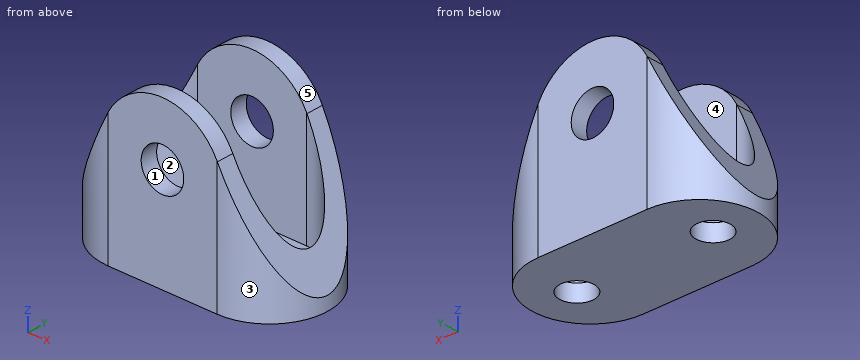
```python
from build123d import *

# Parameters (mm, degrees)
SKETCH1_W          = 44.45
SKETCH1_H          = 31.75
BILLET_DEPTH       = 21.59
SKETCH2_R          = 3.96875
MILL_CUT_1_DEPTH   = 22.59
CUT_EXTRUDE1_DEPTH = 27.305
CUT_EXTRUDE2_DEPTH = 31.48
SKETCH9_R          = 3.175
HOLES_DEPTH        = 4.1750001


with BuildPart() as part:
    # Sketch1 → Billet (new body)
    with BuildSketch(Plane(origin=(0, 0, 0), x_dir=(1, 0, 0), z_dir=(0, 1, 0))):
        Rectangle(SKETCH1_W, SKETCH1_H)
    extrude(amount=BILLET_DEPTH)

    # Sketch2 → Mill Cut 1 (cut, through all)
    with BuildSketch(Plane(origin=(0, 21.59, 0), x_dir=(1, 0, 0), z_dir=(0, 1, 0))):
        with Locations((0, -3.175)):
            Circle(SKETCH2_R)
        with BuildLine():
            Line((-10.236684927, -8.259799082), (-22.225, 15.875))
            Line((-22.225, 15.875), (-22.225, -15.875))
            Line((-22.225, -15.875), (22.225, -15.875))
            Line((22.225, -15.875), (22.225, 15.875))
            Line((22.225, 15.875), (10.236684927, -8.259799082))
            ThreePointArc((10.236684927, -8.259799082), (0, -14.605), (-10.236684927, -8.259799082))
        make_face()
    extrude(amount=-MILL_CUT_1_DEPTH, mode=Mode.SUBTRACT)

    # Sketch6 → Cut-Extrude1 (cut)
    with BuildSketch(Plane(origin=(0, 21.59, 14.605), x_dir=(1, 0, 0), z_dir=(0, 0, 1))):
        with BuildLine():
            Line((-10.16, -3.175), (10.16, -3.175))
            ThreePointArc((10.16, -3.175), (17.78, -10.795), (10.16, -18.415))
            Line((10.16, -18.415), (-10.16, -18.415))
            ThreePointArc((-10.16, -18.415), (-17.78, -10.795), (-10.16, -3.175))
        make_face()
    extrude(amount=-CUT_EXTRUDE1_DEPTH, mode=Mode.SUBTRACT)

    # Sketch8 → Cut-Extrude2 (cut, through all)
    with BuildSketch(Plane(origin=(0, 21.59, 14.605), x_dir=(1, 0, 0), z_dir=(0, 0, 1))):
        with BuildLine():
            Line((-10.16, -21.59), (-60.96, -21.59))
            Line((-60.96, -21.59), (-60.96, 0))
            Line((-60.96, 0), (-10.16, 0))
            ThreePointArc((-10.16, 0), (-20.955, -10.795), (-10.16, -21.59))
        make_face()
    cut_extrude2 = extrude(amount=-CUT_EXTRUDE2_DEPTH, mode=Mode.SUBTRACT)

    # Mirror1: Cut-Extrude2 across plane
    add(cut_extrude2.mirror(Plane(origin=(0, 0, 0), x_dir=(0, 0, 1), z_dir=(1, 0, 0))), mode=Mode.SUBTRACT)

    # Sketch9 → Holes (cut, through all)
    with BuildSketch(Plane.XY.offset(-12.7)):
        with Locations((12.7, 10.795)):
            Circle(SKETCH9_R)
        with Locations((-12.7, 10.795)):
            Circle(SKETCH9_R)
    extrude(amount=-HOLES_DEPTH, mode=Mode.SUBTRACT)


solid = part.part
```
Part model, mm, in its own coordinate system. Face numbers are marked on the shaded views. A direction names the side the tool comes from. Round coordinates to 2 decimals unless told otherwise and drop trailing zeros. Write each loop counter-clockwise with the first axis right and the second up, starting at its lowest first coordinate (ties: lowest second). Pieces come first, ordered by that corner, then holes. Notation, with made-up numbers: (34.5, 51) -> (52.5, 51) arc R22 ccw to (52.5, 83) -> close; hole circle Ø2 at (24.5, 4). An arc over 180 degrees is marked (long way). Return JSON: item names as keys, results as strings. Group by question number.
Q1. Saw through at B-B on y = 10. Write the cut outline in (x, z) (3 decimals).
Q2. Pin check, flat tips, straight feed: pin 1 (2 mm diameter, centred on x = 0.5, z = -10.5, fed in from -Y); pin 2 (4 mm diameter, centred on y = 17.5, z = 4, fed in from +X); pin 3 (6.5 mm diameter, centred on x = 0, z = 3.175, fed in from +Y); pin 4 (4 mm diameter, centred on y = 13, z = -11, fed in from +X). Stop position of each tip, or through.
Q3. Saw through at D-D on z = -10.5. Write the cut outline in (x, y) (3 decimals).
Q4. Saw through at C-C on z = 12. Write the cut outline in (x, y) (3 decimals), plus the area to 3 significant figures.
Q5. Mould opens along Y. For the marked faces 1, 2 and 3 say: pulls with the +Y half, pulls with the -Y half, needs draft (parallel to the pull), parting line crosses it, or undercut.
Q6. Probe L1, parallel to Z at x = 0, y = 20.8 (3 decimals); L2, parallel to Y at x = -3, z = -9.5 (3 decimals); L3, parallel to Z at x = -0.5, y = 16.25 (3 decimals). List the from-to ranges inside material, lowest first. Write a range as [from, to].
Q7. Which spindle directions (+Z, -Z, +X, -X, +Y, -Y) get a long thin tool onto all of the face, cutting with end or side? Do the marked faces 4 and 5. Say none if no direction does.
Q8. Saw through at A-A on x = 12.7. Write the cut outline in (y, z) (3 decimals).
Answer:
{
 "1": {"outline": "(-20.926, -15.875) -> (-15.774, -15.875) -> (-15.774, -12.7) -> (-17.738, -12.7) -> (-17.738, -6.843) -> (-20.926, -13.259) -> close; (-9.626, -15.875) -> (9.626, -15.875) -> (9.626, -12.7) -> (-9.626, -12.7) -> close; (15.774, -15.875) -> (20.926, -15.875) -> (20.926, -13.259) -> (17.738, -6.843) -> (17.738, -12.7) -> (15.774, -12.7) -> close"},
 "2": {"pin 1": "y = 0", "pin 2": "x = 13.34", "pin 3": "through", "pin 4": "x = 20.79"},
 "3": {"outline": "(-19.555, 5.479) arc R10.795 ccw to (-10.16, 0) -> (10.16, 0) arc R10.795 ccw to (19.555, 5.479) -> (19.555, 16.111) arc R10.795 ccw to (10.16, 21.59) -> (-10.16, 21.59) arc R10.795 ccw to (-19.555, 16.111) -> close; hole (-10.16, 3.175) -> (10.16, 3.175) arc R7.62 ccw to (10.16, 18.415) -> (-10.16, 18.415) arc R7.62 ccw to start"},
 "4": {"outline": "(-7.264, 0) -> (7.264, 0) -> (7.264, 3.175) -> (-7.264, 3.175) -> close; (-7.264, 18.415) -> (7.264, 18.415) -> (7.264, 21.59) -> (-7.264, 21.59) -> close", "area": "92.3 mm2"},
 "5": {"face 1": "needs draft", "face 2": "undercut", "face 3": "parting line crosses it"},
 "6": {"L1": "[-15.875, -0.794], [7.144, 14.605]", "L2": "[0, 3.175], [18.415, 21.59]", "L3": "[-15.875, -12.7]"},
 "7": {"face 4": "+Z", "face 5": "+Z, +Y, -Y"},
 "8": {"outline": "(0.303, -15.875) -> (7.62, -15.875) -> (7.62, -12.7) -> (3.611, -12.7) -> (3.611, 3.301) -> (0.303, 3.301) -> close; (13.97, -15.875) -> (21.287, -15.875) -> (21.287, 3.301) -> (17.979, 3.301) -> (17.979, -12.7) -> (13.97, -12.7) -> close"}
}
